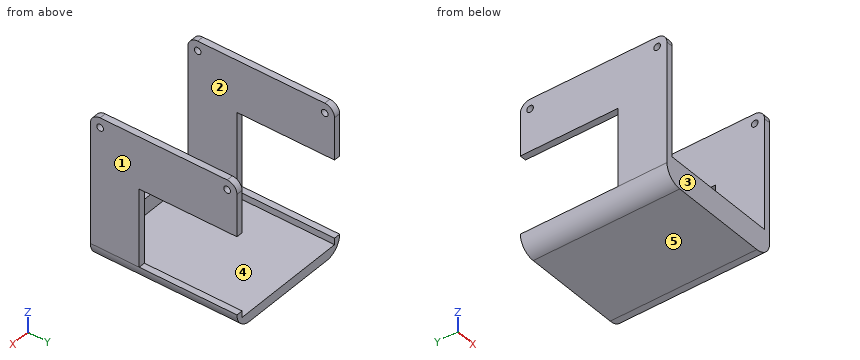
```python
from build123d import *

# Parameters (mm, degrees)
SKETCH_1_W           = 40
SKETCH_1_H           = 45
EXTRUDE_1_DEPTH      = 40
EXTRUDE_1_DEPTH_BACK = 5
SKETCH_2_W           = 36
SKETCH_2_H           = 37
CUT_EXTRUDE_1_DEPTH  = 50
SKETCH_3_R           = 1.025
CUT_EXTRUDE_2_DEPTH  = 2
SKETCH_4_R           = 1.025
CUT_EXTRUDE_3_DEPTH  = 2
SKETCH_5_W           = 36
SKETCH_5_H           = 5
CUT_EXTRUDE_4_DEPTH  = 43
FILLET_6_R           = 5
FILLET_7_R           = 5
FILLET_12_R          = 3
FILLET_13_R          = 3
FILLET_14_R          = 3
FILLET_15_R          = 3
SKETCH_6_W           = 24
SKETCH_6_H           = 30
CUT_EXTRUDE_5_DEPTH  = 44


with BuildPart() as part:
    # 草圖1 → 填料-伸長1 (new body, two sides)
    with BuildSketch(Plane.XY) as extrude_1_sk:
        with Locations((5.454545455, -5.590909091)):
            Rectangle(SKETCH_1_W, SKETCH_1_H)
    extrude(amount=EXTRUDE_1_DEPTH)
    extrude(extrude_1_sk.sketch, amount=-EXTRUDE_1_DEPTH_BACK)

    # 草圖2 → 除料-伸長1 (cut)
    with BuildSketch(Plane(origin=(0, 16.909090909, 0), x_dir=(1, 0, 0), z_dir=(0, 1, 0))):
        with Locations((5.454545455, -21.5)):
            Rectangle(SKETCH_2_W, SKETCH_2_H)
    extrude(amount=-CUT_EXTRUDE_1_DEPTH, mode=Mode.SUBTRACT)

    # 草圖3 → 除料-伸長2 (cut)
    with BuildSketch(Plane.ZY.offset(14.545454545)):
        with Locations((37, -25.090909091)):
            Circle(SKETCH_3_R)
        with Locations((37, 13.909090909)):
            Circle(SKETCH_3_R)
    extrude(amount=-CUT_EXTRUDE_2_DEPTH, mode=Mode.SUBTRACT)

    # 草圖4 → 除料-伸長3 (cut)
    with BuildSketch(Plane(origin=(25.454545455, 0, 0), x_dir=(0, 0, -1), z_dir=(1, 0, 0))):
        with Locations((-37, 13.909090909)):
            Circle(SKETCH_4_R)
        with Locations((-37, -25.090909091)):
            Circle(SKETCH_4_R)
    extrude(amount=-CUT_EXTRUDE_3_DEPTH, mode=Mode.SUBTRACT)

    # 草圖5 → 除料-伸長4 (cut)
    with BuildSketch(Plane(origin=(0, 16.909090909, 0), x_dir=(1, 0, 0), z_dir=(0, 1, 0))):
        with Locations((5.454545455, -0.5)):
            Rectangle(SKETCH_5_W, SKETCH_5_H)
    extrude(amount=-CUT_EXTRUDE_4_DEPTH, mode=Mode.SUBTRACT)

    # 圓角6
    fillet_6_edges = [part.edges().sort_by_distance(p)[0] for p in [
        (-14.545454545, -5.590909091, -5),
    ]]
    fillet(fillet_6_edges, radius=FILLET_6_R)

    # 圓角7
    fillet_7_edges = [part.edges().sort_by_distance(p)[0] for p in [
        (25.454545455, -5.590909091, -5),
    ]]
    fillet(fillet_7_edges, radius=FILLET_7_R)

    # 圓角12
    fillet_12_edges = [part.edges().sort_by_distance(p)[0] for p in [
        (-13.545454545, -28.090909091, 40),
    ]]
    fillet(fillet_12_edges, radius=FILLET_12_R)

    # 圓角13
    fillet_13_edges = [part.edges().sort_by_distance(p)[0] for p in [
        (24.454545455, -28.090909091, 40),
    ]]
    fillet(fillet_13_edges, radius=FILLET_13_R)

    # 圓角14
    fillet_14_edges = [part.edges().sort_by_distance(p)[0] for p in [
        (-13.545454545, 16.909090909, 40),
    ]]
    fillet(fillet_14_edges, radius=FILLET_14_R)

    # 圓角15
    fillet_15_edges = [part.edges().sort_by_distance(p)[0] for p in [
        (24.454545455, 16.909090909, 40),
    ]]
    fillet(fillet_15_edges, radius=FILLET_15_R)

    # 草圖6 → 除料-伸長5 (cut)
    with BuildSketch(Plane.ZY.offset(14.545454545)):
        with Locations((12, 1.909090909)):
            Rectangle(SKETCH_6_W, SKETCH_6_H)
    extrude(amount=-CUT_EXTRUDE_5_DEPTH, mode=Mode.SUBTRACT)


solid = part.part
```
The model under review builds one solid part; all positions refer to its coordinate system, in mm. Face numbers are marked on the shaded views. A direction names the side the tool comes from. Round coordinates to 2 decimals unless told otherwise and drop trailing zeros. Loops run counter-clockwise (first coordinate to the right, second up) from the corner with the lowest first, then second, coordinate; pieces in that order, holes last. Notation, with made-up numbers: (8, 31) -> (47, 31) arc R26 ccw to (47, 66) -> close; hole circle Ø11 at (1, 57.5). An arc over 180 degrees is marked (long way). Answer as a JSON object with one key per item and string values. Group by question number.
1) For the marked faces 4 and 5, list the 3-axis set-ups (+Z, -Z, +X, -X, +Y, -Y) from which the entire face can be reached by the end or side of a thin tool; tool diameter is ignored.
2) Mouldability with a two-part tool opening along X and no side actions: class the marked faces 1, 2 and 3 as released by +X, released by -X, zero draft, split by the parting line, or undercut.
3) We need section B-B on z = 16. Write out the cut boundary in (x, y), then the cut area to 3 significant figures.
4) For line 1 (Y direction, x = 24.2, z = 37); line 2 (X direction, y = -23, z = 37.5); line 3 (Z direction, x = -9, y = -5), list the stretches that pass through material, from the lowest coordinate up. Write a range as [from, to].
5) We need section C-C on y = -16. Write out the cut boundary in (x, z).
6) For pin 1 Ø2 at (x, z) = (-13.5, 10.5) entering from +Y; pin 2 Ø10 at (x, y) = (7.5, 12.5) entering from +Z; pin 3 Ø1.5 at (x, z) = (10.5, -0.5) entering from +Y; pin 4 Ø3.5 at (y, z) = (-25.09, 37) entering from -X, all flat-tipped, find the tip position at first contact; note any pin that passes through.
7) We need section D-D on x = -7.5. Write out the cut boundary in (y, z).
8) We need section A-A on y = 10. Write out the cut boundary in (x, z), then the cut area to 3 significant figures.
Result set:
{
 "1": {"face 4": "+Z, +Y", "face 5": "-Z, +X, -X, +Y, -Y"},
 "2": {"face 1": "released by +X", "face 2": "undercut", "face 3": "zero draft"},
 "3": {"outline": "(-14.55, -28.09) -> (-12.55, -28.09) -> (-12.55, -13.09) -> (-14.55, -13.09) -> close; (23.45, -28.09) -> (25.45, -28.09) -> (25.45, -13.09) -> (23.45, -13.09) -> close", "area": "60.0 mm²"},
 "4": {"line 1": "[-28.09, -26.12], [-24.07, 12.88], [14.93, 16.91]", "line 2": "[-14.55, -12.55], [23.45, 25.45]", "line 3": "[-5, -2]"},
 "5": {"outline": "(-14.55, 0) arc R5 ccw to (-9.55, -5) -> (20.45, -5) arc R5 ccw to (25.45, 0) -> (25.45, 40) -> (23.45, 40) -> (23.45, -2) -> (-12.55, -2) -> (-12.55, 40) -> (-14.55, 40) -> close"},
 "6": {"pin 1": "y = -13.09", "pin 2": "z = -2", "pin 3": "y = -26.09", "pin 4": "x = -14.55"},
 "7": {"outline": "(-28.09, -5) -> (16.91, -5) -> (16.91, -2) -> (-26.09, -2) -> (-26.09, 3) -> (-28.09, 3) -> close"},
 "8": {"outline": "(-14.55, 0) arc R5 ccw to (-9.55, -5) -> (20.45, -5) arc R5 ccw to (25.45, 0) -> (23.45, 0) -> (23.45, -2) -> (-12.55, -2) -> (-12.55, 0) -> close; (-14.55, 24) -> (-12.55, 24) -> (-12.55, 40) -> (-14.55, 40) -> close; (23.45, 24) -> (25.45, 24) -> (25.45, 40) -> (23.45, 40) -> close", "area": "181 mm²"}
}
